Read the model definition and answer for the solid it produces. Units are mm, in the model's axes. Coordinates: 2 decimals unless noted, no trailing zeros. Write each loop counter-clockwise with the first axis right and the second up, starting at its lowest first coordinate (ties: lowest second). Pieces come first, ordered by that corner, then holes. Notation, with made-up numbers: (67, -30) -> (81, -30) arc R14 ccw to (81, -21) -> close; hole circle Ø7 at (86.25, 33). An arc over 180 degrees is marked (long way). One line per item, written item: value. Start each with the question number.
from build123d import *

# Parameters (mm, degrees)
SKETCH1_R           = 4
SKETCH1_R_2         = 1.65
SKETCH1_R_3         = 3.15
SKETCH1_R_4         = 1.5
SKETCH1_R_5         = 11
BOSS_EXTRUDE1_DEPTH = 2


with BuildPart() as part:
    # Sketch1 → Boss-Extrude1 (new body)
    with BuildSketch(Plane.XY):
        with BuildLine():
            ThreePointArc((-137, 0), (-133.485281374, -8.485281374), (-125, -12))
            Line((-125, -12), (125, -12))
            ThreePointArc((125, -12), (133.485281374, -8.485281374), (137, 0))
            Line((137, 0), (137, 180))
            Line((137, 180), (-53.998245329, 180))
            Line((-53.998245329, 180), (-137, 180))
            Line((-137, 180), (-137, 0))
        make_face()
        with Locations((-125, 0)):
            Circle(SKETCH1_R, mode=Mode.SUBTRACT)
        with Locations((-42, 0)):
            Circle(SKETCH1_R, mode=Mode.SUBTRACT)
        with Locations((42, 0)):
            Circle(SKETCH1_R, mode=Mode.SUBTRACT)
        with Locations((57, 8)):
            Circle(SKETCH1_R_2, mode=Mode.SUBTRACT)
        with Locations((57, 28)):
            Circle(SKETCH1_R_2, mode=Mode.SUBTRACT)
        with Locations((77, 8)):
            Circle(SKETCH1_R_2, mode=Mode.SUBTRACT)
        with Locations((97, 8)):
            Circle(SKETCH1_R_2, mode=Mode.SUBTRACT)
        with Locations((125, 0)):
            Circle(SKETCH1_R, mode=Mode.SUBTRACT)
        with Locations((77, 28)):
            Circle(SKETCH1_R_2, mode=Mode.SUBTRACT)
        with Locations((97, 28)):
            Circle(SKETCH1_R_2, mode=Mode.SUBTRACT)
        with Locations((57, 48)):
            Circle(SKETCH1_R_2, mode=Mode.SUBTRACT)
        with Locations((77, 48)):
            Circle(SKETCH1_R_2, mode=Mode.SUBTRACT)
        with Locations((97, 48)):
            Circle(SKETCH1_R_2, mode=Mode.SUBTRACT)
        with Locations((-112.78833811, 103)):
            Circle(SKETCH1_R_3, mode=Mode.SUBTRACT)
        with Locations((-117, 120)):
            Circle(SKETCH1_R_2, mode=Mode.SUBTRACT)
        with Locations((-97, 120)):
            Circle(SKETCH1_R_2, mode=Mode.SUBTRACT)
        with Locations((-77, 120)):
            Circle(SKETCH1_R_2, mode=Mode.SUBTRACT)
        with Locations((-117, 140)):
            Circle(SKETCH1_R_2, mode=Mode.SUBTRACT)
        with Locations((-97, 140)):
            Circle(SKETCH1_R_2, mode=Mode.SUBTRACT)
        with Locations((-77, 140)):
            Circle(SKETCH1_R_2, mode=Mode.SUBTRACT)
        with Locations((-117, 160)):
            Circle(SKETCH1_R_2, mode=Mode.SUBTRACT)
        with Locations((-107, 170)):
            Circle(SKETCH1_R_3, mode=Mode.SUBTRACT)
        with Locations((-97, 160)):
            Circle(SKETCH1_R_2, mode=Mode.SUBTRACT)
        with Locations((-77, 160)):
            Circle(SKETCH1_R_2, mode=Mode.SUBTRACT)
        with Locations((-5, 150)):
            Circle(SKETCH1_R, mode=Mode.SUBTRACT)
        with Locations((24.097224397, 103)):
            Circle(SKETCH1_R_3, mode=Mode.SUBTRACT)
        with Locations((61, 130)):
            Circle(SKETCH1_R_4, mode=Mode.SUBTRACT)
        with Locations((112.15381179, 103)):
            Circle(SKETCH1_R_3, mode=Mode.SUBTRACT)
        with Locations((75, 116)):
            Circle(SKETCH1_R_4, mode=Mode.SUBTRACT)
        with Locations((75, 130)):
            Circle(SKETCH1_R_5, mode=Mode.SUBTRACT)
        with Locations((89, 130)):
            Circle(SKETCH1_R_4, mode=Mode.SUBTRACT)
        with Locations((75, 144)):
            Circle(SKETCH1_R_4, mode=Mode.SUBTRACT)
        with BuildLine():
            ThreePointArc((129, 120), (125, 116), (121, 120))
            Line((121, 120), (121, 170))
            ThreePointArc((121, 170), (125, 174), (129, 170))
            Line((129, 170), (129, 120))
        make_face(mode=Mode.SUBTRACT)
        with Locations((107, 170)):
            Circle(SKETCH1_R_3, mode=Mode.SUBTRACT)
    extrude(amount=BOSS_EXTRUDE1_DEPTH)


solid = part.part
1. A cutting plane is placed at A-A on y = 150. Give the vertices of the cut face in (x, z).
2. A cutting plane is placed at C-C on z = 0.6. Count the separate pieces of the cut face and the enclosed holes in it, then the cut area to 3 significant figures.
3. Find the intervals of material crossed by probe 1 along Y at (x, z) = (-77, 0.9); probe 2 along Y at (x, z) = (75, 1.55); probe 3 along X at (y, z) = (157, 0.7), in increasing order. Write a range as from..to.
4. For a pull along X with two mould halves and no side action, classify faces 1 (the face through (133.39, -8.58, 0.99)), 2 (the face through (-133.58, -8.39, 0.99)), 3 (the face through (-45.2, -2.4, 1)) as +X half, -X half, draft (parallel to the pull), parting line (faces both ways), or undercut.
5. A cutting plane is placed at B-B on x = -5. Give the vertices of the cut face in (y, z).
Derived:
1. outline: (-137, 0) -> (-9, 0) -> (-9, 2) -> (-137, 2) -> close; (-1, 0) -> (121, 0) -> (121, 2) -> (-1, 2) -> close; (129, 0) -> (137, 0) -> (137, 2) -> (129, 2) -> close
2. separate pieces: 1
2. enclosed holes: 34
2. area: 51,100 mm2
3. probe 1: y = -12..118.35, 121.65..138.35, 141.65..158.35, 161.65..180
3. probe 2: y = -12..114.5, 117.5..119, 141..142.5, 145.5..180
3. probe 3: x = -137..121, 129..137
4. face 1: +X half
4. face 2: -X half
4. face 3: undercut
5. outline: (-12, 0) -> (146, 0) -> (146, 2) -> (-12, 2) -> close; (154, 0) -> (180, 0) -> (180, 2) -> (154, 2) -> close
